Check sheet for the modelled part. Datum: model origin and axes. Units: mm. A direction names the side the tool comes from. Give positions to 0.01 mm unless a question says otherwise; leave off trailing zeros. Loops run counter-clockwise (first coordinate to the right, second up) from the corner with the lowest first, then second, coordinate; pieces in that order, holes last. Notation, with made-up numbers: M -0.5,48.5 L 49.5,48.5 A25 ccw 49.5,73.5 Z; hole C 60.25,19 d7. An arc over 180 degrees is marked long. One line per question, with ' | ' between items. Start each with the question number.
from build123d import *

# Parameters (mm, degrees)
F0_W      = 25
F0_H      = 50
F0_R      = 2
F1_DEPTH  = 6
F4_DEPTH  = 10
F6_W      = 20
F6_H      = 50
F7_DEPTH  = 4
F9_W      = 30
F9_H      = 20.7
F10_DEPTH = 1


with BuildPart() as f1:
    # F0 (on Right) → F1 (new body)
    with BuildSketch(Plane.YZ):
        with Locations((6.035548, 17.82273)):
            Rectangle(F0_W, F0_H)
        Circle(F0_R, mode=Mode.SUBTRACT)
        with Locations((6, 35)):
            Circle(F0_R, mode=Mode.SUBTRACT)
    extrude(amount=F1_DEPTH)

    # F3 (on offset) → F4 (join)
    with BuildSketch(Plane.XZ.offset(-14.5)):
        Polygon((93.818079, 27.991471), (3.818079, 27.991471), (3.818079, 19.991471), (73.668075, 19.991471), (93.818079, 19.991471), align=None)
        Polygon((4.434382, -6.643867), (93.818079, 19.991471), (73.668075, 19.991471), (4.434382, -0.639392), align=None)
    extrude(amount=F4_DEPTH)

    # F6 (on offset) → F7 (join)
    with BuildSketch(Plane.XZ.offset(-12.5)):
        with Locations((87.958595, 31.800688)):
            Rectangle(F6_W, F6_H)
    extrude(amount=-F7_DEPTH)

    # F9 (on offset) → F10 (cut)
    with BuildSketch(Plane.XZ.offset(-16.5)):
        with Locations((87.881114, 32.116146)):
            Rectangle(F9_W, F9_H)
    extrude(amount=F10_DEPTH, mode=Mode.SUBTRACT)


solid = f1.part
Q1. Cross-section at B-B (y = 0). Record the cut outline in (x, z), and give its area (3 significant figures).
Q2. Cross-section at D-D (y = 10.75). Record the cut outline in (x, z).
Q3. Material ranges on probe 1 along Z at (x, y) = (2.7, 6); probe 2 along X at (y, z) = (15.5, 15); probe 3 along Z at (x, y) = (82, 15.25), recorded low to high. Write a range as from..to.
Q4. Cross-section at C-C (z = 35). Record the cut outline in (x, y), and give its area (3 significant figures).
Q5. Access from +Z, -Z, +X, -X, +Y, -Y to the whole of each face (thin tool, end or side, straight path). Record for faces 4 (the flat face through (3, 18.536, 17)), 5 (the flat face through (93.818, 9, 24)), 6 (the flat face through (88, 14, 6.801)), 7 (the flat face through (88, 16.5, 14)), 8 (the flat face through (41, 14.5, 23)).
Q6. Cross-section at A-A (y = 6). Record the cut outline in (x, z), and give its area (3 significant figures).
Q7. Depth check by flat-ended pin: P1, Ø10, axis at x = 71.5, y = 15.5, coming from the -Z side; P2, Ø8, axis at x = 43.5, z = 3, coming from the -Y side; P3, Ø4.5, axis at x = 92.5, z = 15.5, coming from the +Y side; P4, Ø1, axis at x = 76, z = 43, coming from the +Y side. Enter the tip coordinate at first touch or a pass-through.
Q8. Draft check along X on faces 1 (the flat face through (51, 10, 27.991)), 2 (the flat face through (0, 6, 18)), 3 (the flat face through (88, 15.5, 32)). Enter one of: released by +X, released by -X, zero draft, split by the parting line, or undercut.
Solved:
1) outline: M 0,-7.18 L 6,-7.18 L 6,-2 L 0,-2 Z; M 0,2 L 6,2 L 6,42.82 L 0,42.82 Z | area: 276 mm²
2) outline: M 0,-7.18 L 6,-7.18 L 6,-6.18 L 93.82,19.99 L 93.82,27.99 L 6,27.99 L 6,42.82 L 0,42.82 Z; hole M 6,-0.17 L 73.67,19.99 L 6,19.99 Z
3) probe 1: z = -7.18..33, 37..42.82 | probe 2: x = 0..6, 77.96..97.96 | probe 3: z = 6.8..56.8
4) outline: M 0,-6.46 L 6,-6.46 L 6,4 L 0,4 Z; M 0,8 L 6,8 L 6,18.54 L 0,18.54 Z; M 77.96,12.5 L 97.96,12.5 L 97.96,15.5 L 77.96,15.5 Z | area: 186 mm²
5) face 4: +Z, -Z, +X, -X, +Y | face 5: +Z, -Z, +X, -Y | face 6: -Z, +X, +Y, -Y | face 7: +Z, -Z, +X, +Y | face 8: +Z, -Z, +Y
6) outline: M 0,-7.18 L 6,-7.18 L 6,-6.18 L 93.82,19.99 L 93.82,27.99 L 6,27.99 L 6,33 L 0,33 Z; M 0,37 L 6,37 L 6,42.82 L 0,42.82 Z; hole M 6,-0.17 L 73.67,19.99 L 6,19.99 Z | area: 1,450 mm²
7) P1: stops at z = 11.88 | P2: stops at y = 4.5 | P3: stops at y = 16.5 | P4: passes through
8) face 1: undercut | face 2: released by -X | face 3: zero draft
